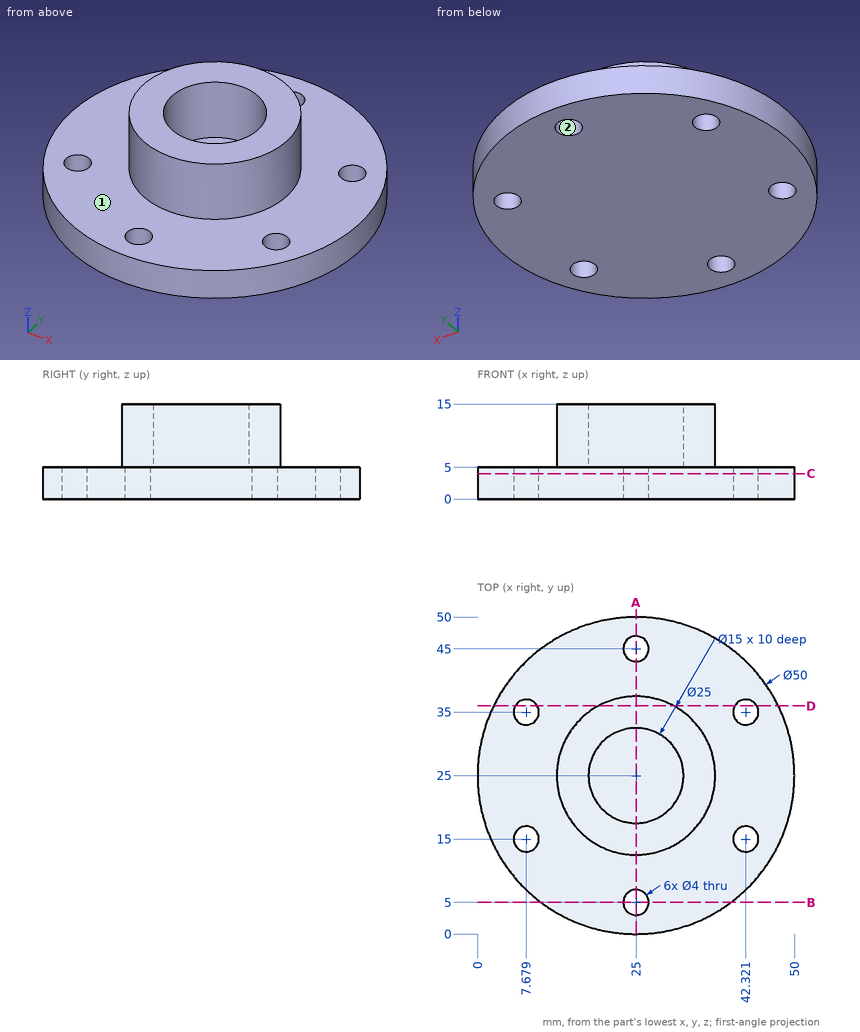
Verification items for this drawing (mm, ordinates from the low corner). A direction names the side the tool comes from. Give positions to 0.01 mm unless a question says otherwise; leave off trailing zeros. Loops run counter-clockwise (first coordinate to the right, second up) from the corner with the lowest first, then second, coordinate; pieces in that order, holes last. Notation, with made-up numbers: M 81,40 L 133,40 A24 ccw 133,78 Z; hole C -13.5,-20.5 d5. An arc over 180 degrees is marked long. Answer as a JSON object with one key per item and string values. Group by question number.
Item 1: Sectioned sample at C-C on z = 4. Record the boundary of the cut face in (x, y).
Item 2: Sectioned sample at D-D on y = 36. Record the boundary of the cut face in (x, z).
Item 3: Sectioned sample at B-B on y = 5. Record the boundary of the cut face in (x, z).
Item 4: Gauge pin test, flat ends, axial feed: pin 1 (2 mm diameter, centred on x = 25, z = 6.5, fed in from -Y); pin 2 (2 mm diameter, centred on x = 14, z = 7.5, fed in from -Y); pin 3 (3 mm diameter, centred on x = 28, z = 13, fed in from +Y); pin 4 (2.5 mm diameter, centred on x = 7.68, y = 35, fed in from +Z). Record the tip position at first contact, or that the pin passes through.
Item 5: Material ranges on L1, parallel to Y at x = 25, z = 3.15; L2, parallel to Y at x = 25, z = 12; L3, parallel to Z at x = 29, y = 47, recorded low to high.
Item 6: Sectioned sample at A-A on x = 25. Record the boundary of the cut face in (y, z).
Item 7: Access from +Z, -Z, +X, -X, +Y, -Y to the whole of each face (thin tool, end or side, straight path). Record for the marked faces 1 and 2.
Findings below:
{
 "1": {"outline": "C 25,25 d50; hole C 7.68,15 d4; hole C 7.68,35 d4; hole C 25,5 d4; hole C 25,45 d4; hole C 42.32,15 d4; hole C 42.32,35 d4"},
 "2": {"outline": "M 2.55,0 L 5.95,0 L 5.95,5 L 2.55,5 Z; M 9.41,0 L 40.59,0 L 40.59,5 L 30.94,5 L 30.94,15 L 19.06,15 L 19.06,5 L 9.41,5 Z; M 44.05,0 L 47.45,0 L 47.45,5 L 44.05,5 Z"},
 "3": {"outline": "M 10,0 L 23,0 L 23,5 L 10,5 Z; M 27,0 L 40,0 L 40,5 L 27,5 Z"},
 "4": {"pin 1": "y = 12.5", "pin 2": "y = 17.5", "pin 3": "y = 37.41", "pin 4": "through"},
 "5": {"L1": "0 to 3, 7 to 43, 47 to 50", "L2": "12.5 to 17.5, 32.5 to 37.5", "L3": "0 to 5"},
 "6": {"outline": "M 0,0 L 3,0 L 3,5 L 0,5 Z; M 7,0 L 43,0 L 43,5 L 37.5,5 L 37.5,15 L 32.5,15 L 32.5,5 L 17.5,5 L 17.5,15 L 12.5,15 L 12.5,5 L 7,5 Z; M 47,0 L 50,0 L 50,5 L 47,5 Z"},
 "7": {"face 1": "+Z", "face 2": "+Z, -Z"}
}
